Autodesk Inventor part; units mm, degrees
ref_plane "YZ Plane" through (0, 0, 0) normal (1, 0, 0) x (0, 1, 0)
ref_plane "XZ Plane" through (0, 0, 0) normal (0, 1, 0) x (-1, 0, 0)
ref_plane "XY Plane" through (0, 0, 0) normal (0, 0, 1) x (1, 0, 0)
sketch "Sketch1" plane through (0, 0, 0) normal (0, 1, 0) x (-1, 0, 0)
  line L0 (8.45, 8.45) -> (-8.45, 8.45)
  line L1 (-8.45, 8.45) -> (-8.45, -8.45)
  line L2 (-8.45, -8.45) -> (8.45, -8.45)
  line L3 (8.45, -8.45) -> (8.45, 8.45)
  point P0 (0, 0)
  dimension "d0" = 16.9
  dimension "d1" = 16.9
  dimension "d2" = 8.45
  dimension "d3" = 8.45
extrude "Extrusion1" add sketch "Sketch1" along normal blind 6.7
fillet "Fillet1" radius 1 4 edges at (8.45, 3.35, -8.45) (8.45, 3.35, 8.45) (-8.45, 3.35, 8.45) (-8.45, 3.35, -8.45)
sketch "Sketch2" plane through (0, 0, 0) normal (0, -1, 0) x (1, 0, 0)
  line L0 (5.95, 8.65) -> (-5.95, 8.65)
  line L1 (-5.95, 8.65) -> (-5.95, 6.55)
  line L2 (-5.95, 6.55) -> (5.95, 6.55)
  line L3 (5.95, 6.55) -> (5.95, 8.65)
  point P0 (0, 0)
  dimension "d7" = 11.9
  dimension "d8" = 5.95
  dimension "d9" = 2.1
  dimension "d10" = 8.65
extrude "Extrusion2" add sketch "Sketch2" along normal blind 0.25 and the other way blind 3.35
mirror "Mirror1" about plane through (0, 0, 0) normal (0, 0, 1) of "Extrusion2"
properties part number "SRP1770TA-101M"
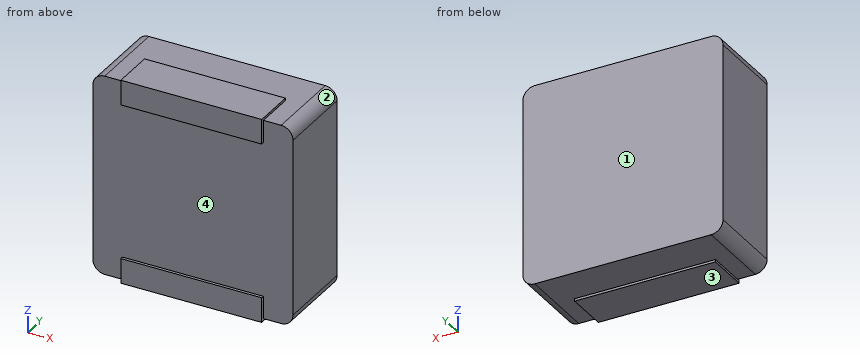
Can you work these out from the model? Positions are in its coordinate system, mm. Face numbers are marked on the shaded views. Coordinates: 2 decimals unless noted, no trailing zeros. Loops run counter-clockwise (first coordinate to the right, second up) from the corner with the lowest first, then second, coordinate; pieces in that order, holes last. Notation, with made-up numbers: M 52,47.25 L 76,47.25 A26 cw 76,69.25 Z; hole C 80.25,70.5 d8. An arc over 180 degrees is marked long. Answer as CSV lines item,"result". Start each with the question number.
1. Suppose I cut it at D-D, the plane x = -7. List the corners of the cut face in (y, z) for me, plus the area to 3 significant figures.
2. Suppose I cut it at B-B, the plane x = -0.5. List the corners of the cut face in (y, z) for me.
3. Suppose I cut it at A-A, the plane y = 5.5. List the corners of the cut face in (x, z) for me, plus the area to 3 significant figures.
4. For pin 1 Ø1 at (x, y) = (3.5, 4) entering from +Z; pin 2 Ø0.6 at (y, z) = (1.5, -8) entering from +X; pin 3 Ø8.5 at (x, z) = (-3, -0.5) entering from -Y, each with a flat end and sliding along its axis, tell me the tip position at first contact or that it passes through.
5. Suppose I cut it at C-C, the plane z = 5.5. List the corners of the cut face in (x, y) for me.
6. Thinking about a two-plate mould opening in Z: for the marked faces 1, 2, 3 and 4, which applies, +Z half, -Z half, draft (parallel to the pull), parting line (faces both ways), or undercut?
7. If I drill on probe 1 along Z at (x, y) = (-1, 5); probe 2 along Y at (x, z) = (-1.25, -3.75), over which ranges is the centre line in solid material (lowest first)? Write a range as [from, to].
Output:
1,outline,"M 0,-8.45 L 6.7,-8.45 L 6.7,8.45 L 0,8.45 Z"
1,area,"113 mm^2"
2,outline,"M -0.25,-8.65 L 3.35,-8.65 L 3.35,-8.45 L 6.7,-8.45 L 6.7,8.45 L 3.35,8.45 L 3.35,8.65 L -0.25,8.65 L -0.25,6.55 L 0,6.55 L 0,-6.55 L -0.25,-6.55 Z"
3,outline,"M -8.45,-7.45 A1 ccw -7.45,-8.45 L 7.45,-8.45 A1 ccw 8.45,-7.45 L 8.45,7.45 A1 ccw 7.45,8.45 L -7.45,8.45 A1 ccw -8.45,7.45 Z"
3,area,"285 mm^2"
4,pin 1,"stops at z = 8.45"
4,pin 2,"stops at x = 8.42"
4,pin 3,"stops at y = 0"
5,outline,"M -8.45,0 L 8.45,0 L 8.45,6.7 L -8.45,6.7 Z"
6,face 1,"draft"
6,face 2,"+Z half"
6,face 3,"-Z half"
6,face 4,"undercut"
7,probe 1,"z = [-8.45, 8.45]"
7,probe 2,"y = [0, 6.7]"
